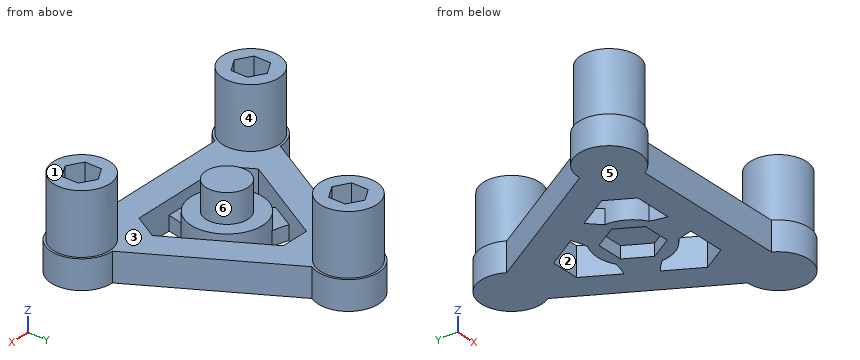
from build123d import *

# Parameters (mm, degrees)
BOSS_EXTRUDE1_DEPTH = 5
BOSS_EXTRUDE2_DEPTH = 5
SKETCH4_R           = 9.75
BOSS_EXTRUDE3_DEPTH = 21
BOSS_EXTRUDE4_START = -5
SKETCH5_R           = 12.441578391
BOSS_EXTRUDE4_DEPTH = 10
SKETCH5_3_R         = 7.25
BOSS_EXTRUDE5_DEPTH = 15
CHAMFER1_SIZE       = 10
CUT_EXTRUDE1_DEPTH  = 10
CUT_EXTRUDE2_DEPTH  = 4.2


with BuildPart() as part:
    # Sketch2 → Boss-Extrude1 (new body, symmetric)
    with BuildSketch(Plane.XY):
        with BuildLine():
            ThreePointArc((8.946673347, 36.860907204), (0, 52.857), (-8.946673347, 36.860907204))
            Line((-8.946673347, 36.860907204), (-36.395818719, -10.682407204))
            ThreePointArc((-36.395818719, -10.682407204), (-45.775504768, -26.4285), (-27.449145372, -26.1785))
            Line((-27.449145372, -26.1785), (27.449145372, -26.1785))
            ThreePointArc((27.449145372, -26.1785), (45.775504768, -26.4285), (36.395818719, -10.682407204))
            Line((36.395818719, -10.682407204), (8.946673347, 36.860907204))
        make_face()
        Polygon((-28.02198399, -16.1785), (0, 32.357), (28.02198399, -16.1785), align=None, mode=Mode.SUBTRACT)
    extrude(amount=BOSS_EXTRUDE1_DEPTH, both=True)

    # Sketch3 → Boss-Extrude2 (add)
    with BuildSketch(Plane.XY):
        with BuildLine():
            Line((-16.510991995, 3.759122981), (-11.510991995, 12.419377019))
            ThreePointArc((-11.510991995, 12.419377019), (0, 10.282645658), (11.510991995, 12.419377019))
            Line((11.510991995, 12.419377019), (16.510991995, 3.759122981))
            ThreePointArc((16.510991995, 3.759122981), (8.905032358, -5.141322829), (5, -16.1785))
            Line((5, -16.1785), (-5, -16.1785))
            ThreePointArc((-5, -16.1785), (-8.905032358, -5.141322829), (-16.510991995, 3.759122981))
        make_face()
    extrude(amount=-BOSS_EXTRUDE2_DEPTH)

    # Sketch4 → Boss-Extrude3 (add)
    with BuildSketch(Plane.XY.offset(5)):
        with Locations((-36.682238028, -21.1785)):
            Circle(SKETCH4_R)
        with Locations((36.682238028, -21.1785)):
            Circle(SKETCH4_R)
        with Locations((0, 42.357)):
            Circle(SKETCH4_R)
    extrude(amount=BOSS_EXTRUDE3_DEPTH)

    # Sketch5 → Boss-Extrude4 (add)
    with BuildSketch(Plane.XY.offset(BOSS_EXTRUDE4_START)):
        Circle(SKETCH5_R)
    extrude(amount=BOSS_EXTRUDE4_DEPTH)

    # Sketch5<3> → Boss-Extrude5 (add)
    with BuildSketch(Plane.XY):
        Circle(SKETCH5_3_R)
    extrude(amount=BOSS_EXTRUDE5_DEPTH)

    # Chamfer1
    chamfer1_edges = [part.edges().sort_by_distance(p)[0] for p in [
        (28.02198399, -16.1785, 0),
        (-28.02198399, -16.1785, 0),
        (0, 32.357, 0),
    ]]
    chamfer(chamfer1_edges, length=CHAMFER1_SIZE)

    # Sketch8 → Cut-Extrude1 (cut)
    with BuildSketch(Plane.XY.offset(26)):
        Polygon((-41.682238028, -24.065251346), (-36.682238028, -26.952002692), (-31.682238028, -24.065251346), (-31.682238028, -18.291748654), (-36.682238028, -15.404997308), (-41.682238028, -18.291748654), align=None)
        Polygon((41.682238028, -24.065251346), (41.682238028, -18.291748654), (36.682238028, -15.404997308), (31.682238028, -18.291748654), (31.682238028, -24.065251346), (36.682238028, -26.952002692), align=None)
        Polygon((0, 48.130502692), (-5, 45.243751346), (-5, 39.470248654), (0, 36.583497308), (5, 39.470248654), (5, 45.243751346), align=None)
    extrude(amount=-CUT_EXTRUDE1_DEPTH, mode=Mode.SUBTRACT)

    # Sketch10 → Cut-Extrude2 (cut)
    with BuildSketch(Plane(origin=(0, 0, -5), x_dir=(-1, 0, 0), z_dir=(0, 0, -1))):
        Polygon((9.381941874, 0), (4.690970937, 8.125), (-4.690970937, 8.125), (-9.381941874, 0), (-4.690970937, -8.125), (4.690970937, -8.125), align=None)
    extrude(amount=-CUT_EXTRUDE2_DEPTH, mode=Mode.SUBTRACT)


solid = part.part
For this review, take the finished solid that the model builds, in its own axes (mm). Face numbers are marked on the shaded views. A direction names the side the tool comes from. Coordinates: 2 decimals unless noted, no trailing zeros. Loops run counter-clockwise (first coordinate to the right, second up) from the corner with the lowest first, then second, coordinate; pieces in that order, holes last. Notation, with made-up numbers: (67, 81.25) - (88, 81.25) arc R19 cw to (88, 106.25) - close; hole circle Ø3 at (48.25, 62). An arc over 180 degrees is marked (long way). Return JSON: item names as keys, results as strings.
Item 1: Take a section at A-A (z = 2.5). Give the boundary of the cut face in (x, y), then the cut area to 3 significant figures.
Determined:
{"outline": "(-36.4, -10.68) arc R10.5 ccw (long way) to (-27.45, -26.18) - (27.45, -26.18) arc R10.5 ccw (long way) to (36.4, -10.68) - (8.95, 36.86) arc R10.5 ccw (long way) to (-8.95, 36.86) - close; circle Ø24.88 at (0, 0); hole (-23.02, -7.52) - (-18.02, -16.18) - (18.02, -16.18) - (23.02, -7.52) - (5, 23.7) - (-5, 23.7) - close", "area": "3,250 mm2"}
Item 2: For the marked faces 1, 2 and 3, list the 3-axis set-ups (+Z, -Z, +X, -X, +Y, -Y) from which the entire face can be reached by the end or side of a thin tool; tool diameter is ignored.
Determined:
{"face 1": "+Z, +X, -X, +Y, -Y", "face 2": "+Z, -Z", "face 3": "+Z"}
Item 3: Take a section at C-C (y = 47). Give the boundary of the cut face in (x, z), then the cut area to 3 significant figures.
Determined:
{"outline": "(-9.42, -5) - (9.42, -5) - (9.42, 5) - (8.57, 5) - (8.57, 26) - (1.96, 26) - (1.96, 16) - (-1.96, 16) - (-1.96, 26) - (-8.57, 26) - (-8.57, 5) - (-9.42, 5) - close", "area": "509 mm2"}
Item 4: Take a section at D-D (x = -38.5). Give the boundary of the cut face in (y, z), then the cut area to 3 significant figures.
Determined:
{"outline": "(-31.52, -5) - (-10.84, -5) - (-10.84, 5) - (-11.6, 5) - (-11.6, 26) - (-16.45, 26) - (-16.45, 16) - (-25.9, 16) - (-25.9, 26) - (-30.76, 26) - (-30.76, 5) - (-31.52, 5) - close", "area": "515 mm2"}
Item 5: Mouldability with a two-part tool opening along X and no side actions: class the marked faces 4, 5 and 6 as pulls with the +X half, pulls with the -X half, needs draft (parallel to the pull), parting line crosses it, or undercut.
Determined:
{"face 4": "undercut", "face 5": "needs draft", "face 6": "parting line crosses it"}
Item 6: For line 1 (Y direction, x = -6.5, z = 4.5); line 2 (X direction, y = -14.5, z = 2.5); line 3 (Z direction, x = 20, y = -24.5), list the stretches that pass through material, from the lowest coordinate up.
Determined:
{"line 1": "y = -26.18 to -16.18, -10.61 to 10.61, 21.1 to 50.6", "line 2": "x = -44.78 to -18.99, 18.99 to 44.78", "line 3": "z = -5 to 5"}
Item 7: Insertion check: pin 1 (1.7 mm diameter, centred on y = -20, z = 19.5, fed in from +X); pin 2 (6.5 mm diameter, centred on y = 42, z = 18.5, fed in from +X); pin 3 (12 mm diameter, centred on y = 35, z = 21.5, fed in from -X). Each pin has a flat end and moves straight along its axis. Give the tip position at first contact, or say it passes through.
Determined:
{"pin 1": "stops at x = 46.43", "pin 2": "stops at x = 9.75", "pin 3": "stops at x = -9.66"}
Item 8: Take a section at B-B (z = 18). State how many separate pieces and enclosed holes the cut face has, then the cut area to 3 significant figures.
Determined:
{"separate pieces": "3", "enclosed holes": "3", "area": "636 mm2"}
